Model file for the job. Use its own axes, mm. Give positions to 0.01 mm unless a question says otherwise; leave off trailing zeros. Order: outer loops, then holes, each group sorted by start corner. A loop starts at its lowest first (then second) coordinate and runs counter-clockwise, first axis right, second up. Notation, with made-up numbers: M 50.5,38.25 L 90.5,38.25 A27 cw 90.5,62.25 Z; hole C -22.75,28 d11. An arc over 180 degrees is marked long. Return JSON: item names as keys, results as strings. Group by question number.
1. Wall check: probe 1 along X at (y, z) = (6.25, 31); probe 2 along Z at (x, y) = (-13.5, 0.5); probe 3 along X at (y, z) = (-9.5, 6). Give the ranges that are in metal, low to high. Write a range as [from, to].
2. Two-plate mould, pull along X, no slides. Class faces 1 (the face through (-13.44, 1.2, 6.15)), 2 (the face through (21, 1, 18)), 3 (the face through (0, 15, 18)): released by +X, released by -X, zero draft, split by the parting line, or undercut.
3. Slice it at D-D on x = 0. List the corners of the cut face in (y, z).
4. Slice it at B-B on y = 0. List the corners of the cut face in (x, z), then the cut area to 3 significant figures.
5. Slice it at C-C on x = -15.25. List the corners of the cut face in (y, z), then the cut area to 3 significant figures.
6. Pin check, flat tips, straight feed: pin 1 (4 mm diameter, centred on x = -11, y = -6, fed in from -Z); pin 2 (2.5 mm diameter, centred on x = -15.25, z = 5, fed in from +Y). Stop position of each tip, or through.
7. Slice it at A-A on z = 5. List the corners of the cut face in (x, y), then the cut area to 3 significant figures.
from build123d import *

# Parameters (mm, degrees)
SKETCH1_W           = 42
SKETCH1_H           = 28
SKETCH1_R           = 6
BOSS_EXTRUDE1_DEPTH = 36
SKETCH2_R           = 2.1463
CUT_EXTRUDE1_DEPTH  = 51.209560843


with BuildPart() as part:
    # Sketch1 → Boss-Extrude1 (new body)
    with BuildSketch(Plane.XY):
        with Locations((0, 1)):
            Rectangle(SKETCH1_W, SKETCH1_H)
        Circle(SKETCH1_R, mode=Mode.SUBTRACT)
    extrude(amount=BOSS_EXTRUDE1_DEPTH)

    # Sketch2 → Cut-Extrude1 (cut, through all)
    with BuildSketch(Plane(origin=(0, 15, 0), x_dir=(1, 0, 0), z_dir=(0, 1, 0))):
        with Locations(Location((-15.25, -5, 0), (0, 0, 270))):
            Circle(SKETCH2_R)
        with Locations(Location((15.25, -5, 0), (0, 0, 270))):
            Circle(SKETCH2_R)
        with Locations(Location((15.25, -31, 0), (0, 0, 270))):
            Circle(SKETCH2_R)
        with Locations(Location((-15.25, -31, 0), (0, 0, 270))):
            Circle(SKETCH2_R)
    extrude(amount=-CUT_EXTRUDE1_DEPTH, mode=Mode.SUBTRACT)


solid = part.part
Result:
{
 "1": {"probe 1": "x = [-21, -17.4], [-13.1, 13.1], [17.4, 21]", "probe 2": "z = [0, 3.76], [6.24, 29.76], [32.24, 36]", "probe 3": "x = [-21, -17.15], [-13.35, 13.35], [17.15, 21]"},
 "2": {"face 1": "undercut", "face 2": "released by +X", "face 3": "zero draft"},
 "3": {"outline": "M -13,0 L -6,0 L -6,36 L -13,36 Z; M 6,0 L 15,0 L 15,36 L 6,36 Z"},
 "4": {"outline": "M -21,0 L -6,0 L -6,36 L -21,36 Z; M 6,0 L 21,0 L 21,36 L 6,36 Z; hole C -15.25,5 d4.29; hole C -15.25,31 d4.29; hole C 15.25,5 d4.29; hole C 15.25,31 d4.29", "area": "1,020 mm2"},
 "5": {"outline": "M -13,0 L 15,0 L 15,2.85 L -13,2.85 Z; M -13,7.15 L 15,7.15 L 15,28.85 L -13,28.85 Z; M -13,33.15 L 15,33.15 L 15,36 L -13,36 Z", "area": "768 mm2"},
 "6": {"pin 1": "stops at z = 0", "pin 2": "passes through"},
 "7": {"outline": "M -21,-13 L -17.4,-13 L -17.4,15 L -21,15 Z; M -13.1,-13 L 13.1,-13 L 13.1,15 L -13.1,15 Z; M 17.4,-13 L 21,-13 L 21,15 L 17.4,15 Z; hole C 0,0 d12", "area": "823 mm2"}
}
